Verification items for the finished model (mm, model axes). Face numbers are marked on the shaded views. A direction names the side the tool comes from. Round coordinates to 2 decimals unless told otherwise and drop trailing zeros. Loops run counter-clockwise (first coordinate to the right, second up) from the corner with the lowest first, then second, coordinate; pieces in that order, holes last. Notation, with made-up numbers: (51.5, 88) - (96.5, 88) arc R16 cw to (96.5, 114) - close; hole circle Ø3 at (19, 17.25). An arc over 180 degrees is marked (long way). Use CSV: the item, a comma, the result in double quotes.
```python
from build123d import *

# Parameters (mm, degrees)
F0_W     = 50.8
F0_H     = 50.8
F1_DEPTH = 50.8
F3_DEPTH = 50.8


with BuildPart() as f1:
    # F0 (on Front) → F1 (new body)
    with BuildSketch(Plane.XZ):
        with Locations((-25.4, 25.4)):
            Rectangle(F0_W, F0_H)
    extrude(amount=F1_DEPTH)

    # F2 (on face) → F3 (cut)
    with BuildSketch(Plane.XZ.offset(50.8)):
        with BuildLine():
            ThreePointArc((-22.619369, 25.4), (-6.474509, 17.005851), (0, 0))
            Line((0, 0), (0, 50.8))
            Line((0, 50.8), (-22.619369, 50.8))
            Line((-22.619369, 50.8), (-22.619369, 25.4))
        make_face()
    extrude(amount=-F3_DEPTH, mode=Mode.SUBTRACT)


solid = f1.part
```
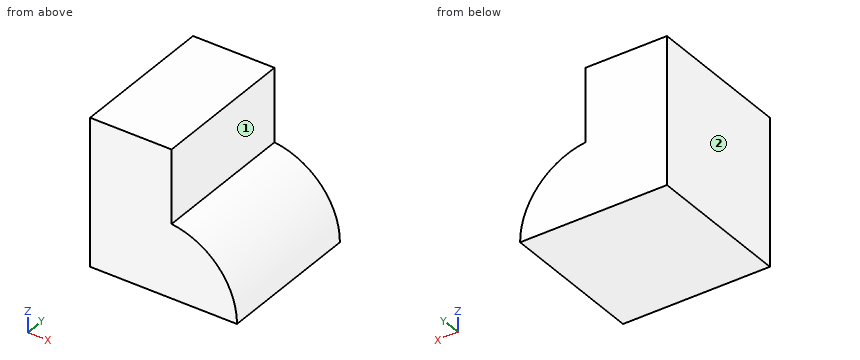
1) Thickness scan on probe 1 along X at (y, z) = (-24, 37); probe 2 along X at (y, z) = (-44.5, 7); probe 3 along Z at (x, y) = (-12, -36). Record the ranges inside material, lowest first. Write a range as [from, to].
Returned:
probe 1,"x = [-50.8, -22.62]"
probe 2,"x = [-50.8, -0.98]"
probe 3,"z = [0, 21.67]"
2) Gauge pin test, flat ends, axial feed: pin 1 Ø12.5 at (y, z) = (-21.5, 44) entering from +X; pin 2 Ø1.5 at (x, y) = (-12.5, -25) entering from +Z; pin 3 Ø6 at (x, z) = (-18, 37.5) entering from +Y. Record the tip position at first contact, or that the pin passes through.
Returned:
pin 1,"stops at x = -22.62"
pin 2,"stops at z = 22.41"
pin 3,"passes through"
3) Cross-section at A-A, the plane y = -12. Record the cut outline in (x, z).
Returned:
outline,"(-50.8, 0) - (0, 0) arc R25.57 ccw to (-22.62, 25.4) - (-22.62, 50.8) - (-50.8, 50.8) - close"
4) Access from +Z, -Z, +X, -X, +Y, -Y to the whole of each face (thin tool, end or side, straight path). Record for the marked faces 1 and 2.
Returned:
face 1,"+Z, +X, +Y, -Y"
face 2,"+Z, -Z, -X, +Y, -Y"
5) Cross-section at C-C, the plane x = -4. Record the cut outline in (y, z), then the cut area to 3 significant figures.
Returned:
outline,"(-50.8, 0) - (0, 0) - (0, 13.73) - (-50.8, 13.73) - close"
area,"698 mm²"
6) Cross-section at B-B, the plane z = 34.5. Record the cut outline in (x, y).
Returned:
outline,"(-50.8, -50.8) - (-22.62, -50.8) - (-22.62, 0) - (-50.8, 0) - close"
